CAD build for the part. Positions are in the model's coordinates, mm. Face numbers are marked on the shaded views. A direction names the side the tool comes from. Give positions to 0.01 mm unless a question says otherwise; leave off trailing zeros. Write each loop counter-clockwise with the first axis right and the second up, starting at its lowest first coordinate (ties: lowest second). Pieces come first, ordered by that corner, then holes. Notation, with made-up numbers: M -22,59 L 21,59 A17 cw 21,76 Z; hole C -9.75,28.5 d1. An arc over 180 degrees is marked long. One line per question, with ' | ' between items. Start each with the question number.
1. Which spindle directions (+Z, -Z, +X, -X, +Y, -Y) get a long thin tool onto all of the face, cutting with end or side? Do the marked faces 1, 2 and 3. Say none if no direction does.
2. Pull direction X, two halves, no side cores. Call the marked faces 4 and 5: released by +X, released by -X, zero draft, split by the parting line, or undercut.
3. Flat gauge pins, fed straight in: pin 1 (3.5 mm diameter, centred on x = 13, y = 10, fed in from -Z); pin 2 (1 mm diameter, centred on x = -12, z = 3, fed in from +Y); pin 3 (1 mm diameter, centred on y = 18, z = -5, fed in from -X). Where does each tip first touch, or does it go through?
4. Cut at B-B, the plane z = -6. Write the cut outline in (x, y).
5. Cut at C-C, the plane x = 2. Write the cut outline in (y, z), then the cut area to 3 significant figures.
6. Wall check: L1, parallel to X at y = 10, z = 4.55; L2, parallel to X at y = 18.25, z = -1.25; L3, parallel to X at y = 7.5, z = -6.25. Give the ranges that are in metal, low to high.
7. Cut at A-A, the plane y = 16. Write the cut outline in (x, z), then the cut area to 3 significant figures.
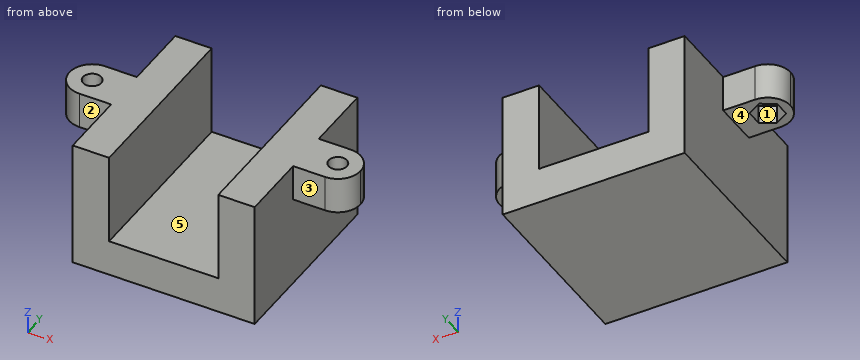
```python
from build123d import *

# Parameters (mm, degrees)
BOSS_EXTRUDE1_DEPTH = 20
SKETCH2_W           = 4
SKETCH2_H           = 12
BOSS_EXTRUDE2_DEPTH = 6
SKETCH3_R           = 1
CUT_EXTRUDE1_DEPTH  = 6
CUT_EXTRUDE2_DEPTH  = 2


with BuildPart() as part:
    # Sketch1 → Boss-Extrude1 (new body)
    with BuildSketch(Plane(origin=(0, 0, 0), x_dir=(1, 0, 0), z_dir=(0, 1, 0))):
        Polygon((-6, -5), (-10, -5), (-10, 9), (10, 9), (10, -5), (6, -5), (6, 5), (-6, 5), align=None)
    extrude(amount=BOSS_EXTRUDE1_DEPTH)

    # Sketch2 → Boss-Extrude2 (add)
    with BuildSketch(Plane(origin=(10, 0, 0), x_dir=(0, 0, -1), z_dir=(1, 0, 0))):
        with Locations((-3, 10)):
            Rectangle(SKETCH2_W, SKETCH2_H)
    boss_extrude2 = extrude(amount=BOSS_EXTRUDE2_DEPTH)

    # Sketch3 → Cut-Extrude1 (cut)
    with BuildSketch(Plane(origin=(0, 0, 1), x_dir=(-1, 0, 0), z_dir=(0, 0, -1))):
        with BuildLine():
            Line((-16, 4), (-10, 4))
            Line((-10, 4), (-10, 7.5))
            Line((-10, 7.5), (-13.5, 7.5))
            ThreePointArc((-13.5, 7.5), (-15.267766953, 8.232233047), (-16, 10))
            Line((-16, 10), (-16, 4))
        make_face()
        with Locations(Location((-13.5, 10, 0), (0, 0, 90))):
            Circle(SKETCH3_R)
        with BuildLine():
            Line((-16, 16), (-16, 10))
            ThreePointArc((-16, 10), (-15.267766953, 11.767766953), (-13.5, 12.5))
            Line((-13.5, 12.5), (-10, 12.5))
            Line((-10, 12.5), (-10, 16))
            Line((-10, 16), (-16, 16))
        make_face()
    cut_extrude1 = extrude(amount=-CUT_EXTRUDE1_DEPTH, mode=Mode.SUBTRACT)

    # Sketch4 → Cut-Extrude2 (cut)
    with BuildSketch(Plane(origin=(0, 0, 1), x_dir=(-1, 0, 0), z_dir=(0, 0, -1))):
        Polygon((-13.5, 11.75), (-15.015544457, 10.875), (-15.015544457, 9.125), (-13.5, 8.25), (-11.984455543, 9.125), (-11.984455543, 10.875), align=None)
    cut_extrude2 = extrude(amount=-CUT_EXTRUDE2_DEPTH, mode=Mode.SUBTRACT)

    # Mirror1: Boss-Extrude2, Cut-Extrude1, Cut-Extrude2 across plane
    add(boss_extrude2.mirror(Plane(origin=(0, 0, 0), x_dir=(0, 0, 1), z_dir=(1, 0, 0))))
    add(cut_extrude1.mirror(Plane(origin=(0, 0, 0), x_dir=(0, 0, 1), z_dir=(1, 0, 0))), mode=Mode.SUBTRACT)
    add(cut_extrude2.mirror(Plane(origin=(0, 0, 0), x_dir=(0, 0, 1), z_dir=(1, 0, 0))), mode=Mode.SUBTRACT)


solid = part.part
```
Here are the results:
1) face 1: -Z | face 2: +Z, -Z, -X, -Y | face 3: +Z, -Z, +X, -Y
2) face 4: zero draft | face 5: undercut
3) pin 1: z = 1 | pin 2: y = 12.5 | pin 3: x = -10
4) outline: M -10,0 L 10,0 L 10,20 L -10,20 Z
5) outline: M 0,-9 L 20,-9 L 20,-5 L 0,-5 Z | area: 80.0 mm^2
6) L1: -16 to -14.5, -12.5 to -6, 6 to 12.5, 14.5 to 16 | L2: -10 to -6, 6 to 10 | L3: -10 to 10
7) outline: M -10,-9 L 10,-9 L 10,5 L 6,5 L 6,-5 L -6,-5 L -6,5 L -10,5 Z | area: 160 mm^2
